Can you work these out from the model? Positions are in its coordinate system, mm. A direction names the side the tool comes from. Give positions to 0.01 mm unless a question says otherwise; leave off trailing zeros. Order: outer loops, then holes, each group sorted by start corner. A loop starts at its lowest first (then second) coordinate and runs counter-clockwise, first axis right, second up.
Item 1: I'm going to push flat-ended pins straight in: pin 1 Ø0.6 at (y, z) = (-13, -1.5) entering from +X; pin 2 Ø1 at (x, z) = (23.5, -0.5) entering from -Y. Where does each tip first touch, or does it pass through?
Item 2: Which directions (+Z, -Z, +X, -X, +Y, -Y) give clear straight access to the entire face, cutting with the end or side of a thin tool? Please do faces 5 (the flat face through (-15, 33, -1)), 6 (the flat face through (-34, -25, -1)), 7 (the flat face through (34, -5, -1)).
Item 3: If we mould it in two halves opening along Y, with no side actions, what happens to faces 1 (the flat face through (34, -25, -1)), 2 (the flat face through (0, 35, -1)), 3 (the flat face through (-34, 25, -1)), 4 (the flat face through (25, 34, -1))? For each: +Y half, -Y half, draft (parallel to the pull), parting line (faces both ways), or undercut.
Item 4: I want a section at A-A, the plane x = 10. Write out the boundary of the cut face in (y, z).
Item 5: If I drill on line 1 along Y through (x, z) = (-7, -1.5), over which ranges is the centre line in solid material (lowest first)?
```python
from build123d import *

# Parameters (mm, degrees)
SKETCH1_W           = 70
SKETCH1_H           = 70
BOSS_EXTRUDE1_DEPTH = 2
SKETCH2_W           = 2
SKETCH2_H           = 20
SKETCH2_W_2         = 20
SKETCH2_H_2         = 2
CUT_EXTRUDE1_DEPTH  = 2


with BuildPart() as part:
    # Sketch1 → Boss-Extrude1 (new body)
    with BuildSketch(Plane.XY):
        Rectangle(SKETCH1_W, SKETCH1_H)
    extrude(amount=-BOSS_EXTRUDE1_DEPTH)

    # Sketch2 → Cut-Extrude1 (cut)
    with BuildSketch(Plane.XY):
        with Locations((-34, 15)):
            Rectangle(SKETCH2_W, SKETCH2_H)
        with Locations((-34, -15)):
            Rectangle(SKETCH2_W, SKETCH2_H)
        with Locations((-15, -34)):
            Rectangle(SKETCH2_W_2, SKETCH2_H_2)
        with Locations((15, -34)):
            Rectangle(SKETCH2_W_2, SKETCH2_H_2)
        with Locations((34, -15)):
            Rectangle(SKETCH2_W, SKETCH2_H)
        with Locations((34, 15)):
            Rectangle(SKETCH2_W, SKETCH2_H)
        with Locations((15, 34)):
            Rectangle(SKETCH2_W_2, SKETCH2_H_2)
        with Locations((-15, 34)):
            Rectangle(SKETCH2_W_2, SKETCH2_H_2)
    extrude(amount=-CUT_EXTRUDE1_DEPTH, mode=Mode.SUBTRACT)


solid = part.part
```
Results list:
1. pin 1: stops at x = 33
1. pin 2: stops at y = -33
2. face 5: +Z, -Z, +Y
2. face 6: +Z, -Z, -X
2. face 7: +Z, -Z, +X
3. face 1: undercut
3. face 2: +Y half
3. face 3: undercut
3. face 4: draft
4. outline: (-33, -2) - (33, -2) - (33, 0) - (-33, 0) - close
5. line 1: y = -33 to 33
